```python
from build123d import *

# Parameters (mm, degrees)
BOSS_EXTRUDE1_DEPTH = 762
BOSS_EXTRUDE2_START = -762
BOSS_EXTRUDE2_DEPTH = 1524


with BuildPart() as part:
    # Sketch1 → Boss-Extrude1 (new, symmetric)
    with BuildSketch(Plane.XY):
        Polygon((3.175, 2.54), (-1.905, 2.54), (-1.905, -2.54), (3.175, -2.54), (3.175, -18.415), (-3.175, -18.415), (-3.175, 18.415), (3.175, 18.415), align=None)
    extrude(amount=BOSS_EXTRUDE1_DEPTH, both=True)

    # Sketch2 → Boss-Extrude2 (add)
    with BuildSketch(Plane.XY.offset(BOSS_EXTRUDE2_START)):
        Polygon((-3.175, 18.415), (-3.175, -18.415), (-9.669122699, -18.415), align=None)
    extrude(amount=BOSS_EXTRUDE2_DEPTH)


solid = part.part
```
Here's how the part is built. I have some questions about the finished solid (model axes, mm). Give positions to 0.01 mm unless a question says otherwise; leave off trailing zeros. Loops run counter-clockwise (first coordinate to the right, second up) from the corner with the lowest first, then second, coordinate; pieces in that order, holes last. Notation, with made-up numbers: (-39.75, 3.5) -> (5.25, 3.5) arc R16 cw to (5.25, 25.5) -> close; hole circle Ø11 at (-32, 25.5). An arc over 180 degrees is marked (long way). Use one line per item in the form item = value. Start each with the question number.
1) Imagine slicing it at B-B (z = 266). Please give me the cut outline in (x, y) (3 decimals).
2) Please list where these lines run through material, in increasing order: line 1 along Y through (x, z) = (-1.25, -641.5) (3 decimals); line 2 along X through (y, z) = (14.5, -206) (3 decimals); line 3 along X through (y, z) = (11, 459) (3 decimals).
3) Imagine slicing it at A-A (x = 0.25). Please give me the cut outline in (y, z) (3 decimals), then the cut area to 3 significant figures.
4) Imagine slicing it at C-C (y = -12). Please give me the cut outline in (x, z) (3 decimals).
5) For P1, Ø12, axis at y = -10.5, z = 18, coming from the -X side; P2, Ø1.5, axis at y = 1, z = 178, coming from the +X side (3 decimals), each with a flat end and sliding along its axis, tell me the tip position at first contact or that it passes through.
Check values:
q1.outline = (-9.669, -18.415) -> (3.175, -18.415) -> (3.175, -2.54) -> (-1.905, -2.54) -> (-1.905, 2.54) -> (3.175, 2.54) -> (3.175, 18.415) -> (-3.175, 18.415) -> close
q2.line_1 = -18.415 to -2.54, 2.54 to 18.415
q2.line_2 = -3.865 to 3.175
q2.line_3 = -4.482 to 3.175
q3.outline = (-18.415, -762) -> (-2.54, -762) -> (-2.54, 762) -> (-18.415, 762) -> close; (2.54, -762) -> (18.415, -762) -> (18.415, 762) -> (2.54, 762) -> close
q3.area = 48,400 mm^2
q4.outline = (-8.538, -762) -> (3.175, -762) -> (3.175, 762) -> (-8.538, 762) -> close
q5.P1 = -9.33
q5.P2 = -1.905
